```python
from build123d import *

# Parameters (mm, degrees)
BOSS_EXTRUDE1_DEPTH = 1.5
FILLET1_R           = 5
FILLET3_R           = 7
FILLET4_R           = 2
FILLET5_R           = 5


with BuildPart() as part:
    # Sketch1 → Boss-Extrude1 (new, symmetric)
    with BuildSketch(Plane(origin=(0, 0, 0), x_dir=(1, 0, 0), z_dir=(0, 1, 0))):
        with BuildLine():
            Line((0, 33.06), (0, 0))
            Line((0, 0), (14.8, 0))
            Line((14.8, 0), (14.8, 9.13))
            ThreePointArc((14.8, 9.13), (16.3, 10.63), (17.8, 9.13))
            Line((17.8, 9.13), (17.8, 0))
            Line((17.8, 0), (28.82, 0))
            Line((28.82, 0), (40.93, 25.6))
            Line((40.93, 25.6), (23.039915269, 25.6))
            ThreePointArc((23.039915269, 25.6), (21.54, 27.084056775), (23.00803062, 28.599661085))
            Line((23.00803062, 28.599661085), (30.66, 28.762351413))
            Line((30.66, 28.762351413), (39.893121089, 57.462102219))
            ThreePointArc((39.893121089, 57.462102219), (44.38174059, 58.083541414), (48.292108688, 60.373282238))
            Line((48.292108688, 60.373282238), (41.74, 61.438906704))
            ThreePointArc((41.74, 61.438906704), (40.500247088, 63.160247088), (42.221587473, 64.4))
            Line((42.221587473, 64.4), (50.522210261, 63.05))
            ThreePointArc((50.522210261, 63.05), (52.200549071, 69.291091406), (50.287964746, 75.464426347))
            Line((50.287964746, 75.464426347), (48.619556224, 70.509026223))
            ThreePointArc((48.619556224, 70.509026223), (46.719339491, 69.566064737), (45.776378004, 71.466281471))
            Line((45.776378004, 71.466281471), (47.986855886, 78.031701286))
            ThreePointArc((47.986855886, 78.031701286), (47.402242068, 78.484891921), (46.79, 78.9))
            Line((46.79, 78.9), (34.22, 83.484702826))
            Line((34.22, 83.484702826), (20.171354305, 41.75831525))
            ThreePointArc((20.171354305, 41.75831525), (18.405987937, 38.194020326), (15.753217128, 35.230319303))
            ThreePointArc((15.753217128, 35.230319303), (15.499590166, 41.461362705), (13.089045589, 47.212841067))
            ThreePointArc((13.089045589, 47.212841067), (10.959051171, 52.738918493), (11.232947268, 58.654946626))
            ThreePointArc((11.232947268, 58.654946626), (10.606012481, 59.845600176), (9.361365657, 59.334173363))
            ThreePointArc((9.361365657, 59.334173363), (7.842242616, 53.86210101), (8.259081404, 48.198395856))
            ThreePointArc((8.259081404, 48.198395856), (7.08728895, 39.015533985), (0, 33.06))
        make_face()
    extrude(amount=BOSS_EXTRUDE1_DEPTH, both=True)

    # Fillet1
    fillet1_edges = [part.edges().sort_by_distance(p)[0] for p in [
        (40.93, 0, -25.6),
    ]]
    fillet(fillet1_edges, radius=FILLET1_R)

    # Fillet3
    fillet3_edges = [part.edges().sort_by_distance(p)[0] for p in [
        (34.22, 0, -83.484702826),
    ]]
    fillet(fillet3_edges, radius=FILLET3_R)

    # Fillet4
    fillet4_edges = [part.edges().sort_by_distance(p)[0] for p in [
        (0, 0, 0),
    ]]
    fillet(fillet4_edges, radius=FILLET4_R)

    # Fillet5
    fillet5_edges = [part.edges().sort_by_distance(p)[0] for p in [
        (28.82, 0, 0),
    ]]
    fillet(fillet5_edges, radius=FILLET5_R)


solid = part.part
```
Could you check a few things on this model? Use its own coordinates, in mm. A direction names the side the tool comes from. Round coordinates to 2 decimals unless told otherwise and drop trailing zeros. Loops run counter-clockwise (first coordinate to the right, second up) from the corner with the lowest first, then second, coordinate; pieces in that order, holes last. Notation, with made-up numbers: M 27,52 L 51,52 A20 ccw 51,64 Z; hole C 28,-8 d10. An arc over 180 degrees is marked long. Put each result on its own line as item: value.
Q1. Imagine slicing it at A-A (z = -49.5). Write out the boundary of the cut face in (x, y), then the cut area to 3 significant figures.
Check result:
outline: M 7.99,-1.5 L 11.88,-1.5 L 11.88,1.5 L 7.99,1.5 Z; M 22.78,-1.5 L 37.33,-1.5 L 37.33,1.5 L 22.78,1.5 Z
area: 55.3 mm2
Q2. Imagine slicing it at C-C (z = -27.1). Write out the boundary of the cut face in (x, y), then the cut area to 3 significant figures.
Check result:
outline: M 0,-1.5 L 21.54,-1.5 L 21.54,1.5 L 0,1.5 Z
area: 64.6 mm2
Q3. On a 3-axis mill with a long thin cutter (end or side, diameter ignored), from which of +Z, -Z, +X, -X, +Y, -Y can I reach the whole of each face in a straight line? I mean faces 4 (the face through (17.8, 0, -5)), 5 (the face through (35.21, 0.02, -42.91)), 6 (the face through (46.314, 0.021, -63.734)). Say none if no direction works.
Check result:
face 4: +Z, +Y, -Y
face 5: +X, +Y, -Y
face 6: +Y, -Y
Q4. Imagine slicing it at D-D (x = 17). Write out the boundary of the cut face in (y, z).
Check result:
outline: M -1.5,-36.43 L 1.5,-36.43 L 1.5,-10.46 L -1.5,-10.46 Z
Q5. For pin 1 (1.5 mm diameter, centred on y = 0.5, z = -3, fed in from +X); pin 2 (8 mm diameter, centred on x = 28.5, z = -70.5, fed in from +Y), each with a flat end and sliding along its axis, tell me the tip position at first contact or that it passes through.
Check result:
pin 1: x = 30.59
pin 2: y = 1.5
Q6. I need wall thicknesses on probe 1 along X at (y, z) = (1.1, -75); probe 2 along X at (y, z) = (-0.7, -74); probe 3 along X at (y, z) = (-1.1, -26). Which ranges of each line are inside material? Lowest first, please.
Check result:
probe 1: 31.36 to 46.97, 50.13 to 50.58
probe 2: 31.03 to 46.63, 49.79 to 51.11
probe 3: 0 to 22.02
Q7. Thinking about a two-plate mould opening in Z: for faces 1 (the face through (7.15, 0.02, -39.13)), 2 (the face through (0.57, 0.02, -0.6)), 3 (the face through (26.133, 0.021, -59.465)), which applies, released by +Z, released by -Z, zero draft, split by the parting line, or undercut?
Check result:
face 1: undercut
face 2: released by +Z
face 3: released by -Z
